Here's how the part is built. I have some questions about the finished solid (model axes, mm). Face numbers are marked on the shaded views. Give positions to 0.01 mm unless a question says otherwise; leave off trailing zeros. Loops run counter-clockwise (first coordinate to the right, second up) from the corner with the lowest first, then second, coordinate; pieces in that order, holes last.
Q1. Thinking about a two-plate mould opening in Y: for the marked faces 1, 2 and 3, which applies, pulls with the +Y half, pulls with the -Y half, needs draft (parallel to the pull), parting line crosses it, or undercut?
Q2. Suppose I cut it at B-B (y = -27). List the corners of the cut face in (x, z) for me, and give its area (3 significant figures).
Q3. Suppose I cut it at D-D (y = 0). Count the separate pieces of the cut face and the enclosed holes in it, and give its area (3 significant figures).
Q4. Suppose I cut it at A-A (x = 0). List the corners of the cut face in (y, z) for me.
Q5. I need wall thicknesses on probe 1 along Y at (x, z) = (0, -7.8); probe 2 along Y at (x, z) = (-1, -19.5); probe 3 along Y at (x, z) = (30, -5.75) (3 decimals). Which ranges of each line are inside material? Lowest first, please.
Q6. Suppose I cut it at C-C (x = -33). List the corners of the cut face in (y, z) for me, and give its area (3 significant figures).
Q7. I'm going to push flat-ended pins straight in: P1, Ø5, axis at y = -14.5, z = -5.5, coming from the -X side; P2, Ø6.5, axis at x = 7, y = 1, coming from the +Z side; P3, Ø7.5, axis at x = 8, y = 0, coming from the -Z side; P4, Ø2, axis at x = 30, y = 0, coming from the -Z side. Where does each tip first touch, or does it pass through?
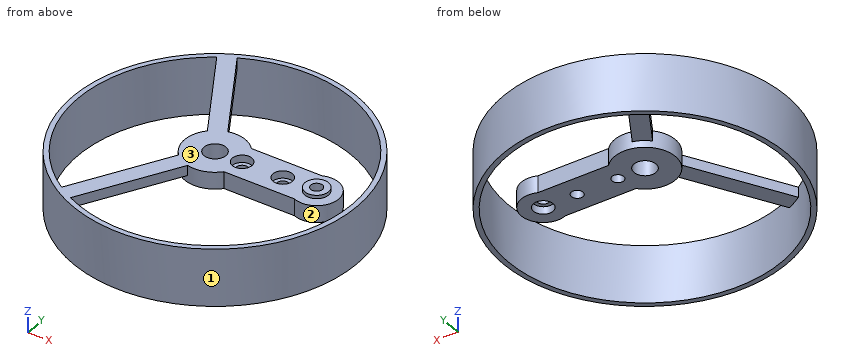
```python
from build123d import *

# Parameters (mm, degrees)
BOSS_EXTRUDE1_START     = -9
SKETCH1_W               = 30
SKETCH1_H               = 12
BOSS_EXTRUDE1_DEPTH     = 5
BOSS_EXTRUDE2_START     = -9
SKETCH2_R               = 9
BOSS_EXTRUDE2_DEPTH     = 5
BOSS_EXTRUDE3_START     = -9
SKETCH3_R               = 6.5
BOSS_EXTRUDE3_DEPTH     = 5
CUT_EXTRUDE1_DEPTH      = 39.655530005
CUT_EXTRUDE1_DEPTH_BACK = 39.655530005
SKETCH4_R               = 3.25
CUT_EXTRUDE2_DEPTH      = 39.655530005
CUT_EXTRUDE2_DEPTH_BACK = 39.655530005
SKETCH5_R               = 1.725
CUT_EXTRUDE3_START      = -6.2
SKETCH6_R               = 2.9
CUT_EXTRUDE3_DEPTH      = 2.2
CUT_EXTRUDE4_START      = -6.2
SKETCH7_R               = 2.9
CUT_EXTRUDE4_DEPTH      = 2.2
CUT_EXTRUDE5_START      = -9
SKETCH8_R               = 2.9
CUT_EXTRUDE5_DEPTH      = 2.2
BOSS_EXTRUDE4_START     = -4
SKETCH9_R               = 3.5
BOSS_EXTRUDE4_DEPTH     = 1
CUT_EXTRUDE6_DEPTH      = 39.655530005
CUT_EXTRUDE6_DEPTH_BACK = 39.655530005
SKETCH10_R              = 1.725
BOSS_EXTRUDE5_START     = -21
SKETCH11_R              = 42
SKETCH11_R_2            = 40.5
BOSS_EXTRUDE5_DEPTH     = 17
BOSS_EXTRUDE6_START     = -7
BOSS_EXTRUDE6_DEPTH     = 3


with BuildPart() as part:
    # Sketch1 → Boss-Extrude1 (new body)
    with BuildSketch(Plane.XY.offset(BOSS_EXTRUDE1_START)):
        with Locations((15, 0)):
            Rectangle(SKETCH1_W, SKETCH1_H)
    extrude(amount=BOSS_EXTRUDE1_DEPTH)

    # Sketch2 → Boss-Extrude2 (add)
    with BuildSketch(Plane.XY.offset(BOSS_EXTRUDE2_START)):
        Circle(SKETCH2_R)
    extrude(amount=BOSS_EXTRUDE2_DEPTH)

    # Sketch3 → Boss-Extrude3 (add)
    with BuildSketch(Plane.XY.offset(BOSS_EXTRUDE3_START)):
        with Locations((30, 0)):
            Circle(SKETCH3_R)
    extrude(amount=BOSS_EXTRUDE3_DEPTH)

    # Sketch4 → Cut-Extrude1 (cut, two sides: drawn at the far end of the back side and taken through both)
    with BuildSketch(Plane.XY.offset(-CUT_EXTRUDE1_DEPTH_BACK)):
        Circle(SKETCH4_R)
    extrude(amount=CUT_EXTRUDE1_DEPTH + CUT_EXTRUDE1_DEPTH_BACK, mode=Mode.SUBTRACT)

    # Sketch5 → Cut-Extrude2 (cut, two sides: drawn at the far end of the back side and taken through both)
    with BuildSketch(Plane.XY.offset(-CUT_EXTRUDE2_DEPTH_BACK)):
        with Locations((8, 0)):
            Circle(SKETCH5_R)
        with Locations((20, 0)):
            Circle(SKETCH5_R)
        with Locations((30, 0)):
            Circle(SKETCH5_R)
    extrude(amount=CUT_EXTRUDE2_DEPTH + CUT_EXTRUDE2_DEPTH_BACK, mode=Mode.SUBTRACT)

    # Sketch6 → Cut-Extrude3 (cut)
    with BuildSketch(Plane.XY.offset(CUT_EXTRUDE3_START)):
        with Locations((8, 0)):
            Circle(SKETCH6_R)
    extrude(amount=CUT_EXTRUDE3_DEPTH, mode=Mode.SUBTRACT)

    # Sketch7 → Cut-Extrude4 (cut)
    with BuildSketch(Plane.XY.offset(CUT_EXTRUDE4_START)):
        with Locations((20, 0)):
            Circle(SKETCH7_R)
    extrude(amount=CUT_EXTRUDE4_DEPTH, mode=Mode.SUBTRACT)

    # Sketch8 → Cut-Extrude5 (cut)
    with BuildSketch(Plane.XY.offset(CUT_EXTRUDE5_START)):
        with Locations((30, 0)):
            Circle(SKETCH8_R)
    extrude(amount=CUT_EXTRUDE5_DEPTH, mode=Mode.SUBTRACT)

    # Sketch9 → Boss-Extrude4 (add)
    with BuildSketch(Plane.XY.offset(BOSS_EXTRUDE4_START)):
        with Locations((30, 0)):
            Circle(SKETCH9_R)
    extrude(amount=BOSS_EXTRUDE4_DEPTH)

    # Sketch10 → Cut-Extrude6 (cut, two sides: drawn at the far end of the back side and taken through both)
    with BuildSketch(Plane.XY.offset(-CUT_EXTRUDE6_DEPTH_BACK)):
        with Locations((30, 0)):
            Circle(SKETCH10_R)
    extrude(amount=CUT_EXTRUDE6_DEPTH + CUT_EXTRUDE6_DEPTH_BACK, mode=Mode.SUBTRACT)



with BuildPart() as body_2:
    # Sketch11 → Boss-Extrude5 (new body)
    with BuildSketch(Plane.XY.offset(BOSS_EXTRUDE5_START)):
        Circle(SKETCH11_R)
        Circle(SKETCH11_R_2, mode=Mode.SUBTRACT)
    extrude(amount=BOSS_EXTRUDE5_DEPTH)


with BuildPart() as part_1:
    add(part.part)

    add(body_2.part)  # Boss-Extrude6 merges body 2
    # Sketch12 → Boss-Extrude6 (add)
    with BuildSketch(Plane.XY.offset(BOSS_EXTRUDE6_START)):
        Polygon((-1.334936491, 7.312177826), (-18.584936491, 37.190054257), (-22.915063509, 34.690054257), (-5.665063509, 4.812177826), align=None)
        Polygon((-5.665063509, -4.812177826), (-22.915063509, -34.690054257), (-18.584936491, -37.190054257), (-1.334936491, -7.312177826), align=None)
    extrude(amount=BOSS_EXTRUDE6_DEPTH)


solid = part_1.part
```
Solutions:
1. face 1: parting line crosses it
1. face 2: undercut
1. face 3: needs draft
2. outline: (-32.17, -21) - (-30.19, -21) - (-30.19, -4) - (-32.17, -4) - close; (-18.48, -7) - (-12.7, -7) - (-12.7, -4) - (-18.48, -4) - close; (30.19, -21) - (32.17, -21) - (32.17, -4) - (30.19, -4) - close
2. area: 84.8 mm2
3. separate pieces: 7
3. enclosed holes: 0
3. area: 182 mm2
4. outline: (-42, -21) - (-40.5, -21) - (-40.5, -4) - (-42, -4) - close; (-9, -9) - (-3.25, -9) - (-3.25, -4) - (-9, -4) - close; (3.25, -9) - (9, -9) - (9, -4) - (3.25, -4) - close; (40.5, -21) - (42, -21) - (42, -4) - (40.5, -4) - close
5. probe 1: y = -42 to -40.5, -9 to -3.25, 3.25 to 9, 40.5 to 42
5. probe 2: y = -41.99 to -40.49, 40.49 to 41.99
5. probe 3: y = -29.394 to -27.208, -6.5 to -1.725, 1.725 to 6.5, 27.208 to 29.394
6. outline: (-25.98, -21) - (-23.48, -21) - (-23.48, -4) - (-25.98, -4) - close; (23.48, -21) - (25.98, -21) - (25.98, -4) - (23.48, -4) - close
6. area: 85.1 mm2
7. P1: stops at x = -40.25
7. P2: stops at z = -4
7. P3: stops at z = -9
7. P4: passes through
